Input: part model. Units: mm. Frame: model coordinates. Round coordinates to 2 decimals unless told otherwise and drop trailing zeros. Loops run counter-clockwise (first coordinate to the right, second up) from the corner with the lowest first, then second, coordinate; pieces in that order, holes last.
(1) Cut plane A-A, the plane x = 2.5. Output: boundary loops of the cut face in (y, z), and give its area (4 significant figures).
(2) Cut plane B-B, the plane y = 48. Output: boundary loops of the cut face in (x, z), and give its area (3 significant figures).
(3) Draft query along X for faces 1 (the face through (-65.16, 49.52, 0.74)), 2 (the face through (-1, 1, 1.5)). Return one class per face: released by +X, released by -X, zero draft, split by the parting line, or undercut.
(4) Cut plane C-C, the plane x = -63.5. Output: boundary loops of the cut face in (y, z).
(5) First-contact query: pin 1 Ø2.5 at (x, y) = (-63.5, 13) entering from -Z; pin 2 Ø5 at (x, y) = (-63.5, -50) entering from -Z. Flat tips, straight axial feed; report the tip coordinate or a pass-through.
(6) Line query: line 1 (Y direction, x = -63.5, z = 1.25); line 2 (Y direction, x = 67.5, z = 1.2); line 3 (X direction, y = -3, z = 0.45). Output: solid intervals per line, ascending.
from build123d import *

# Parameters (mm, degrees)
SKETCH_1_W      = 145
SKETCH_1_H      = 130
SKETCH_1_R      = 2.25
SKETCH_1_R_2    = 2.75
EXTRUDE_1_DEPTH = 1.5


with BuildPart() as part:
    # Эскиз1 → Вытянуть1 (new body)
    with BuildSketch(Plane.XY):
        Rectangle(SKETCH_1_W, SKETCH_1_H)
        with Locations((-67.5, 60)):
            Circle(SKETCH_1_R, mode=Mode.SUBTRACT)
        with Locations(Location((-67.5, -60, 0), (0, 0, 180))):
            Circle(SKETCH_1_R, mode=Mode.SUBTRACT)
        with Locations((67.5, -60)):
            Circle(SKETCH_1_R, mode=Mode.SUBTRACT)
        with Locations(Location((67.5, 60, 0), (0, 0, 180))):
            Circle(SKETCH_1_R, mode=Mode.SUBTRACT)
        with Locations((-63.5, -2)):
            Circle(SKETCH_1_R, mode=Mode.SUBTRACT)
        with Locations(Location((-63.5, -50, 0), (0, 0, 180))):
            Circle(SKETCH_1_R, mode=Mode.SUBTRACT)
        with Locations((2.5, -2)):
            Circle(SKETCH_1_R, mode=Mode.SUBTRACT)
        with Locations(Location((2.5, -50, 0), (0, 0, 180))):
            Circle(SKETCH_1_R, mode=Mode.SUBTRACT)
        with Locations((40.5, 0)):
            Circle(SKETCH_1_R_2, mode=Mode.SUBTRACT)
        with Locations((-63.5, 13)):
            Circle(SKETCH_1_R, mode=Mode.SUBTRACT)
        with Locations((-63.5, 48)):
            Circle(SKETCH_1_R, mode=Mode.SUBTRACT)
        with Locations((-3.5, 13)):
            Circle(SKETCH_1_R, mode=Mode.SUBTRACT)
        with Locations((-3.5, 48)):
            Circle(SKETCH_1_R, mode=Mode.SUBTRACT)
    extrude(amount=EXTRUDE_1_DEPTH)


solid = part.part
Reported:
1. outline: (-65, 0) - (-52.25, 0) - (-52.25, 1.5) - (-65, 1.5) - close; (-47.75, 0) - (-4.25, 0) - (-4.25, 1.5) - (-47.75, 1.5) - close; (0.25, 0) - (65, 0) - (65, 1.5) - (0.25, 1.5) - close
1. area: 181.5 mm2
2. outline: (-72.5, 0) - (-65.75, 0) - (-65.75, 1.5) - (-72.5, 1.5) - close; (-61.25, 0) - (-5.75, 0) - (-5.75, 1.5) - (-61.25, 1.5) - close; (-1.25, 0) - (72.5, 0) - (72.5, 1.5) - (-1.25, 1.5) - close
2. area: 204 mm2
3. face 1: undercut
3. face 2: zero draft
4. outline: (-65, 0) - (-52.25, 0) - (-52.25, 1.5) - (-65, 1.5) - close; (-47.75, 0) - (-4.25, 0) - (-4.25, 1.5) - (-47.75, 1.5) - close; (0.25, 0) - (10.75, 0) - (10.75, 1.5) - (0.25, 1.5) - close; (15.25, 0) - (45.75, 0) - (45.75, 1.5) - (15.25, 1.5) - close; (50.25, 0) - (65, 0) - (65, 1.5) - (50.25, 1.5) - close
5. pin 1: passes through
5. pin 2: stops at z = 0
6. line 1: y = -65 to -52.25, -47.75 to -4.25, 0.25 to 10.75, 15.25 to 45.75, 50.25 to 65
6. line 2: y = -65 to -62.25, -57.75 to 57.75, 62.25 to 65
6. line 3: x = -72.5 to -65.52, -61.48 to 0.48, 4.52 to 72.5
